For this review, take the finished solid that the model builds, in its own axes (mm). A direction names the side the tool comes from. Coordinates: 2 decimals unless noted, no trailing zeros. Loops run counter-clockwise (first coordinate to the right, second up) from the corner with the lowest first, then second, coordinate; pieces in that order, holes last. Notation, with made-up numbers: M 50.25,-32 L 94.25,-32 A6 ccw 94.25,-25 Z; hole C -4,-8 d2. An arc over 180 degrees is marked long. Put each result on its own line as item: value.
Autodesk Inventor part; units mm, degrees
ref_plane "YZ Plane" through (0, 0, 0) normal (1, 0, 0) x (0, 1, 0)
ref_plane "XZ Plane" through (0, 0, 0) normal (0, 1, 0) x (-1, 0, 0)
ref_plane "XY Plane" through (0, 0, 0) normal (0, 0, 1) x (1, 0, 0)
sketch "Esboço1" plane through (0, 0, 0) normal (0, 1, 0) x (-1, 0, 0)
  line L0 (19.6154, -5.2564) -> (-20.3846, -5.2564)
  line L1 (-20.3846, -5.2564) -> (-20.3846, -105.2564)
  line L2 (-20.3846, -105.2564) -> (19.6154, -105.2564)
  line L3 (19.6154, -105.2564) -> (19.6154, -5.2564)
  point P0 (0, 0)
  dimension "d0" = 40
  dimension "d4" = 100
extrude "Extrusão1" add sketch "Esboço1" along normal blind 20
sketch "Esboço2" plane through (0, 20, 0) normal (0, 1, 0) x (1, 0, 0)
  circle A0 centre (0, 55.2564) radius 12.5
  circle A1 centre (0, 55.2564) radius 11
  line L0 (20.3846, 105.2564) -> (-19.6154, 105.2564)
  point P0 (0, 0)
  dimension "d11" = 22
  dimension "d12" = 25
  dimension "d13" = 50
extrude "Extrusão2" add sketch "Esboço2" along normal blind 7
sketch "Esboço3" plane through (0, 0, 0) normal (0, -1, 0) x (1, 0, 0)
  circle A0 centre (0.3846, -25.2576) radius 2.5
  circle A1 centre (0, -85.2564) radius 2.5
  line L0 (20.3846, -105.2564) -> (-19.6154, -105.2564)
  line L1 (20.3846, -5.2564) -> (20.3846, -105.2564)
  point P0 (0, 0)
  dimension "d16" = 5
  dimension "d17" = 5
  dimension "d18" = 60
  dimension "d19" = 20
  dimension "d20" = 20
extrude "Extrusão3" add sketch "Esboço3" along normal blind 5
properties part number "Suporte para estrutura_CPY" material "ABS plástico"
(1) For pin 1 (5 mm diameter, centred on x = -2, z = -56, fed in from +Y); pin 2 (1.5 mm diameter, centred on y = -1.5, z = -26, fed in from +X); pin 3 (4 mm diameter, centred on x = -14.5, z = -75, fed in from -Y), all flat-tipped, find the tip position at first contact; note any pin that passes through.
Determined:
pin 1: stops at y = 20
pin 2: stops at x = 2.88
pin 3: stops at y = 0
(2) Add section C-C (y = 22.5). Write out the cut boundary in (x, z), plus the area to 3 significant figures.
Determined:
outline: C 0,-55.26 d25; hole C 0,-55.26 d22
area: 111 mm^2
(3) Add section B-B (z = -33). Write out the cut boundary in (x, y), plus the area to 3 significant figures.
Determined:
outline: M -19.62,0 L 20.38,0 L 20.38,20 L -19.62,20 Z
area: 800 mm^2
(4) Tool access review of faces 1 (the cylindrical face through (-8.107, 23.451, -47.822)), 2 (the cylindrical face through (1.54, -2.46, -23.04)), 3 (the flat face through (0, 10, -5.256)): name each direction out of +Z, -Z, +X, -X, +Y, -Y from which nothing blocks a thin tool from reaching the whole face with its end or side.
Determined:
face 1: +Y
face 2: -Y
face 3: +Z, +X, -X, +Y, -Y
(5) Add section A-A (x = 0). Write out the cut boundary in (y, z), plus the area to 3 significant figures.
Determined:
outline: M -5,-87.76 L 0,-87.76 L 0,-105.26 L 20,-105.26 L 20,-67.76 L 27,-67.76 L 27,-66.26 L 20,-66.26 L 20,-44.26 L 27,-44.26 L 27,-42.76 L 20,-42.76 L 20,-5.26 L 0,-5.26 L 0,-22.79 L -5,-22.79 L -5,-27.73 L 0,-27.73 L 0,-82.76 L -5,-82.76 Z
area: 2,070 mm^2
(6) Draft analysis for pull direction X (two halves, no side actions). For faces 4 (the cylindrical face through (6.72, 23.451, -44.716)), 5 (the flat face through (1, 0, -55)), 6 (the flat face through (0, 20, -55)), 7 (the flat face through (-19.615, 10, -56)), state which applies: +X half, -X half, draft (parallel to the pull), parting line (faces both ways), or undercut.
Determined:
face 4: parting line
face 5: draft
face 6: undercut
face 7: -X half
(7) Add section D-D (x = -9). Write out the cut boundary in (y, z), plus the area to 3 significant figures.
Determined:
outline: M 0,-105.26 L 20,-105.26 L 20,-63.93 L 27,-63.93 L 27,-61.58 L 20,-61.58 L 20,-48.93 L 27,-48.93 L 27,-46.58 L 20,-46.58 L 20,-5.26 L 0,-5.26 Z
area: 2,030 mm^2
(8) Wall thickness on line 1 along Z through (x, y) = (0, 22); line 2 along Y through (x, z) = (4.5, -56); line 3 along Z through (x, y) = (4, 22): over which ranges is each line inside the solid? List them lowest first. Write a range as [from, to].
Determined:
line 1: z = [-67.76, -66.26], [-44.26, -42.76]
line 2: y = [0, 20]
line 3: z = [-67.1, -65.5], [-45.01, -43.41]
